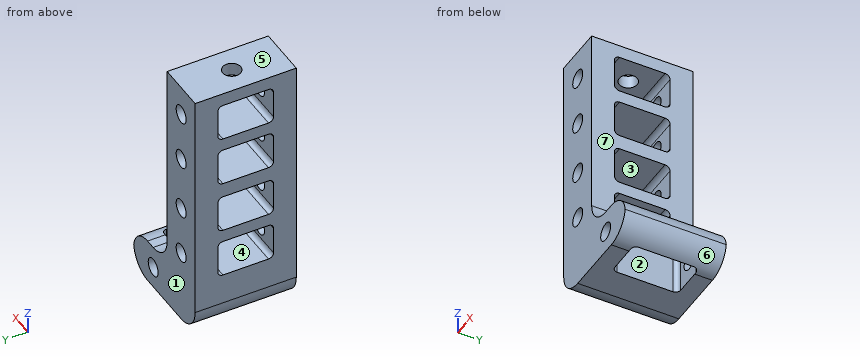
from build123d import *

# Parameters (mm, degrees)
F1_DEPTH      = 20
F0_R          = 1.778
F3_DEPTH      = 25
F3_DEPTH_BACK = 25
F5_DEPTH      = 25
F5_DEPTH_BACK = 25
F6_R          = 1.778
F7_DEPTH      = 2.611541214
F8_R          = 1.778
F9_DEPTH      = 5


with BuildPart() as f1:
    # F0 (on Front) → F1 (new body)
    with BuildSketch(Plane.XZ):
        with BuildLine():
            ThreePointArc((22, -3.7987752631), (21.9909406431, -4.0996265512), (21.963795401, -4.3993876316))
            ThreePointArc((21.963795401, -4.3993876316), (21.9909406431, -4.6991487119), (22, -5))
            Line((22, -5), (22, -3.7987752631))
        make_face()
    extrude(amount=F1_DEPTH)


with BuildPart() as f1b:
    # F0 (on Front) → F1, piece 2 (new body)
    with BuildSketch(Plane.XZ):
        with BuildLine():
            Line((10, 43), (0, 43))
            Line((0, 43), (0, 0))
            Line((0, 0), (0, -3.7987752631))
            ThreePointArc((0, -3.7987752631), (1.4644660941, -7.3343091691), (5, -8.7987752631))
            Line((5, -8.7987752631), (17, -8.7987752631))
            ThreePointArc((17, -8.7987752631), (20.3163939873, -7.5406372222), (21.963795401, -4.3993876316))
            ThreePointArc((21.963795401, -4.3993876316), (20.3163939873, -1.2581380409), (17, 0))
            Line((17, 0), (15, 0))
            ThreePointArc((15, 0), (11.4644660941, 1.4644660941), (10, 5))
            Line((10, 5), (10, 43))
        make_face()
        with Locations((5, 5.9739946499)):
            Circle(F0_R, mode=Mode.SUBTRACT)
        with Locations((5, 15.9739946499)):
            Circle(F0_R, mode=Mode.SUBTRACT)
        with Locations((15, -4.4229245409)):
            Circle(F0_R, mode=Mode.SUBTRACT)
        with Locations((5, 26.9999946499)):
            Circle(F0_R, mode=Mode.SUBTRACT)
        with Locations((5, 36.9999946499)):
            Circle(F0_R, mode=Mode.SUBTRACT)
    extrude(amount=F1_DEPTH)

    # F2 (on face) → F3 (cut, two sides)
    with BuildSketch(Plane.YZ.offset(10)) as f3_sk:
        with BuildLine():
            ThreePointArc((-15.5, 3.430458786), (-15.2071067812, 2.7233520048), (-14.5, 2.430458786))
            Line((-14.5, 2.430458786), (-5.5, 2.430458786))
            ThreePointArc((-5.5, 2.430458786), (-4.7928932188, 2.7233520048), (-4.5, 3.430458786))
            Line((-4.5, 3.430458786), (-4.5, 8.930458786))
            ThreePointArc((-4.5, 8.930458786), (-4.7928932188, 9.6375655672), (-5.5, 9.930458786))
            Line((-5.5, 9.930458786), (-14.5, 9.930458786))
            ThreePointArc((-14.5, 9.930458786), (-15.2071067812, 9.6375655672), (-15.5, 8.930458786))
            Line((-15.5, 8.930458786), (-15.5, 3.430458786))
        make_face()
        with BuildLine():
            Line((-5.5, 19.930458786), (-14.5, 19.930458786))
            ThreePointArc((-14.5, 19.930458786), (-15.2071067812, 19.6375655672), (-15.5, 18.930458786))
            Line((-15.5, 18.930458786), (-15.5, 13.430458786))
            ThreePointArc((-15.5, 13.430458786), (-15.2071067812, 12.7233520048), (-14.5, 12.430458786))
            Line((-14.5, 12.430458786), (-5.5, 12.430458786))
            ThreePointArc((-5.5, 12.430458786), (-4.7928932188, 12.7233520048), (-4.5, 13.430458786))
            Line((-4.5, 13.430458786), (-4.5, 18.930458786))
            ThreePointArc((-4.5, 18.930458786), (-4.7928932188, 19.6375655672), (-5.5, 19.930458786))
        make_face()
        with BuildLine():
            ThreePointArc((-14.5, 40.388458786), (-15.2071067812, 40.0955655672), (-15.5, 39.388458786))
            Line((-15.5, 39.388458786), (-15.5, 33.888458786))
            ThreePointArc((-15.5, 33.888458786), (-15.2071067812, 33.1813520048), (-14.5, 32.888458786))
            Line((-14.5, 32.888458786), (-5.5, 32.888458786))
            ThreePointArc((-5.5, 32.888458786), (-4.7928932188, 33.1813520048), (-4.5, 33.888458786))
            Line((-4.5, 33.888458786), (-4.5, 39.388458786))
            ThreePointArc((-4.5, 39.388458786), (-4.7928932188, 40.0955655672), (-5.5, 40.388458786))
            Line((-5.5, 40.388458786), (-14.5, 40.388458786))
        make_face()
        with BuildLine():
            ThreePointArc((-14.5, 30.388458786), (-15.2071067812, 30.0955655672), (-15.5, 29.388458786))
            Line((-15.5, 29.388458786), (-15.5, 23.888458786))
            ThreePointArc((-15.5, 23.888458786), (-15.2071067812, 23.1813520048), (-14.5, 22.888458786))
            Line((-14.5, 22.888458786), (-5.5, 22.888458786))
            ThreePointArc((-5.5, 22.888458786), (-4.7928932188, 23.1813520048), (-4.5, 23.888458786))
            Line((-4.5, 23.888458786), (-4.5, 29.388458786))
            ThreePointArc((-4.5, 29.388458786), (-4.7928932188, 30.0955655672), (-5.5, 30.388458786))
            Line((-5.5, 30.388458786), (-14.5, 30.388458786))
        make_face()
    extrude(amount=-F3_DEPTH, mode=Mode.SUBTRACT)
    extrude(f3_sk.sketch, amount=F3_DEPTH_BACK, mode=Mode.SUBTRACT)

    # F4 (on face) → F5 (cut, two sides)
    with BuildSketch(Plane.XY) as f5_sk:
        with BuildLine():
            Line((11.963795401, -16.5), (17.463795401, -16.5))
            ThreePointArc((17.463795401, -16.5), (18.1709021822, -16.2071067812), (18.463795401, -15.5))
            Line((18.463795401, -15.5), (18.463795401, -4.5))
            ThreePointArc((18.463795401, -4.5), (18.1709021822, -3.7928932188), (17.463795401, -3.5))
            Line((17.463795401, -3.5), (11.963795401, -3.5))
            ThreePointArc((11.963795401, -3.5), (11.2566886198, -3.7928932188), (10.963795401, -4.5))
            Line((10.963795401, -4.5), (10.963795401, -15.5))
            ThreePointArc((10.963795401, -15.5), (11.2566886198, -16.2071067812), (11.963795401, -16.5))
        make_face()
    extrude(amount=-F5_DEPTH, mode=Mode.SUBTRACT)
    extrude(f5_sk.sketch, amount=F5_DEPTH_BACK, mode=Mode.SUBTRACT)

    # F6 (on face) → F7 (join, through all)
    with BuildSketch(Plane.XY.offset(43)):
        with Locations((5, -13.5)):
            Circle(F6_R)
        with Locations((5, -6.5)):
            Circle(F6_R)
    extrude(amount=-F7_DEPTH)

    # F8 (on face) → F9 (cut)
    with BuildSketch(Plane.XY.offset(43)):
        with Locations((5, -10)):
            Circle(F8_R)
    extrude(amount=-F9_DEPTH, mode=Mode.SUBTRACT)


solid = f1b.part
Input: part model. Units: mm. Frame: model coordinates. Face numbers are marked on the shaded views. A direction names the side the tool comes from. Give positions to 0.01 mm unless a question says otherwise; leave off trailing zeros. Write each loop counter-clockwise with the first axis right and the second up, starting at its lowest first coordinate (ties: lowest second). Pieces come first, ordered by that corner, then holes.
Q1. Section D-D, the plane y = -18. Output: boundary loops of the cut face in (x, z).
Q2. Section C-C, the plane x = 16. Output: boundary loops of the cut face in (y, z).
Q3. First-contact query: P1, Ø4, axis at x = 13.5, z = 32, coming from the +Y side; P2, Ø3, axis at x = 5, y = -10, coming from the +Z side; P3, Ø1.5, axis at y = -12.5, z = 10, coming from the +X side; P4, Ø2, axis at x = 16.5, y = -1.5, coming from the +Z side. Flat tips, straight axial feed; report the tip coordinate or a pass-through.
Q4. Section A-A, the plane y = -13. Output: boundary loops of the cut face in (x, z).
Q5. Material intervals for probe 1 along Z at (x, y) = (7.75, -12.5); probe 2 along Z at (x, y) = (5, -2.05); probe 3 along Z at (x, y) = (6.25, -10.25), sorted ascending.
Q6. Section B-B, the plane y = -10. State how many separate pieces and enclosed holes the cut face has, plus the area to 3 significant figures.
Q7. Pull-direction query (Z, two-part tool) for the marked faces 4, 5, 6 and 7; classes: pulls with the +Z half, pulls with the -Z half, needs draft (parallel to the pull), parting line crosses it, or undercut.
Q8. Set-up query: the marked faces 1, 2 and 3. Return all of +Z, -Z, +X, -X, +Y, -Y with unobstructed straight access to the full face (end or side cutting, diameter ignored); none if empty.
Filled in:
1. outline: (0, -3.8) arc R5 ccw to (5, -8.8) - (17, -8.8) arc R5 ccw to (21.96, -4.4) arc R5 ccw to (17, 0) - (15, 0) arc R5 cw to (10, 5) - (10, 43) - (0, 43) - close; hole circle Ø3.56 at (5, 5.97); hole circle Ø3.56 at (5, 15.97); hole circle Ø3.56 at (5, 27); hole circle Ø3.56 at (5, 37); hole circle Ø3.56 at (15, -4.42)
2. outline: (-20, -8.8) - (-16.5, -8.8) - (-16.5, -5.89) - (-20, -5.89) - close; (-20, -2.95) - (-16.5, -2.95) - (-16.5, 0) - (-20, 0) - close; (-3.5, -8.8) - (0, -8.8) - (0, -5.89) - (-3.5, -5.89) - close; (-3.5, -2.95) - (0, -2.95) - (0, 0) - (-3.5, 0) - close
3. P1: passes through
3. P2: stops at z = 32.89
3. P3: stops at x = 10
3. P4: stops at z = 0
4. outline: (0, -3.8) arc R5 ccw to (5, -8.8) - (10.96, -8.8) - (10.96, 2.05) arc R5 cw to (10.71, 2.43) - (0, 2.43) - close; (0, 9.93) - (10, 9.93) - (10, 12.43) - (0, 12.43) - close; (0, 19.93) - (10, 19.93) - (10, 22.89) - (0, 22.89) - close; (0, 30.39) - (10, 30.39) - (10, 32.89) - (0, 32.89) - close; (0, 40.39) - (10, 40.39) - (10, 43) - (0, 43) - close; (18.46, -8.58) arc R5 ccw to (21.96, -4.4) arc R5 ccw to (18.46, -0.22) - close
5. probe 1: z = -8.8 to 2.43, 9.93 to 12.43, 19.93 to 22.89, 30.39 to 32.89, 40.39 to 43
5. probe 2: z = -8.8 to 4.2, 7.75 to 14.2, 17.75 to 25.22, 28.78 to 35.22, 38.78 to 43
5. probe 3: z = -8.8 to 2.43, 9.93 to 12.43, 19.93 to 22.89, 30.39 to 32.89
6. separate pieces: 7
6. enclosed holes: 0
6. area: 235 mm2
7. face 4: undercut
7. face 5: pulls with the +Z half
7. face 6: pulls with the -Z half
7. face 7: needs draft
8. face 1: +Z, -Z, +X, -X, +Y
8. face 2: +Z, -Z
8. face 3: +X, -X
